Part model, mm, in its own coordinate system. A direction names the side the tool comes from. Coordinates: 2 decimals unless noted, no trailing zeros. Write each loop counter-clockwise with the first axis right and the second up, starting at its lowest first coordinate (ties: lowest second). Pieces come first, ordered by that corner, then holes. Notation, with made-up numbers: (6, -21.5) -> (10, -21.5) arc R16 ccw to (10, -1.5) -> close; hole circle Ø1 at (-33, -38.75). An arc over 180 degrees is marked (long way). One line per question, with ' | ' between items. Start each with the question number.
Item 1: Saw through at A-A (x = -82.5). List the corners of the cut face in (y, z), and give its area (3 significant figures).
Item 2: 3-axis set-ups, long thin cutter, end or side, ignore diameter. For faces 5 (the flat face through (-40, 42, 8)), 6 (the flat face through (40, 42, 8)), 7 (the cylindrical face through (88.849, 0.132, 3.254)), 8 (the flat face through (-1, 43, 15)): which of +Z, -Z, +X, -X, +Y, -Y reach the whole face in a straight line?
Item 3: Saw through at C-C (z = 12.5). Count the separate pieces of the cut face and the enclosed holes in it, and give its area (3 significant figures).
Item 4: Two-plate mould, pull along X, no slides. Class faces 1 (the flat face through (72, 0, 20)), 2 (the flat face through (-1, 0, 19.5)), 3 (the cylindrical face through (-85.8, 5.1, 13.4)), 4 (the flat face through (-105, 0, 10)): pulls with the +X half, pulls with the -X half, needs draft (parallel to the pull), parting line crosses it, or undercut.
Item 5: Saw through at D-D (x = 44). List the corners of the cut face in (y, z), and give its area (3 significant figures).
Item 6: Saw through at B-B (y = -6.5). List the corners of the cut face in (x, z).
Item 7: Pin check, flat tips, straight feed: pin 1 (13 mm diameter, centred on x = -82.5, y = 5, fed in from -Z); pin 2 (12 mm diameter, centred on y = 45.5, z = 6, fed in from -X); pin 3 (6.5 mm diameter, centred on x = -23, y = 6.5, fed in from +Z); pin 4 (21 mm diameter, centred on x = 82.5, y = 5, fed in from +Z). Stop position of each tip, or through.
Item 8: Probe probe 1 along Y at (x, z) = (82.5, 14.5); probe 2 along Y at (x, z) = (-25, 5.25); probe 3 along Y at (x, z) = (82.5, 1.5). List the from-to ranges inside material, lowest first. Write a range as [from, to].
from build123d import *

# Parameters (mm, degrees)
SKETCH1_W                                      = 210
SKETCH1_H                                      = 50
EXTRUDE1_DEPTH                                 = 20
CBORE_FOR_M6_HEX_HEAD_FLANGE_BOLT1_D           = 6.6
CBORE_FOR_M6_HEX_HEAD_FLANGE_BOLT1_CBORE_D     = 16
CBORE_FOR_M6_HEX_HEAD_FLANGE_BOLT1_CBORE_DEPTH = 6.6
CUT_EXTRUDE1_REACH                             = 52
SKETCH4_W                                      = 80
SKETCH4_H                                      = 0.5
M6_TAPPED_HOLE1_D                              = 5
SKETCH7_W                                      = 80
SKETCH7_H                                      = 35
EXTRUDE2_DEPTH                                 = 19.5
SKETCH8_W                                      = 80
SKETCH8_H                                      = 5
CUT_EXTRUDE2_DEPTH                             = 35
M6_TAPPED_HOLE2_D                              = 5


with BuildPart() as part:
    # Sketch1 → Extrude1 (new body)
    with BuildSketch(Plane.XY):
        Rectangle(SKETCH1_W, SKETCH1_H)
    extrude(amount=EXTRUDE1_DEPTH)

    # CBORE for M6 Hex Head Flange Bolt1 (through all)
    with Locations(Plane(origin=(0, 0, 0), x_dir=(-1, 0, 0), z_dir=(0, 0, -1))):
        with Locations((82.5, 5), (-82.5, 5)):
            CounterBoreHole(CBORE_FOR_M6_HEX_HEAD_FLANGE_BOLT1_D / 2, CBORE_FOR_M6_HEX_HEAD_FLANGE_BOLT1_CBORE_D / 2, CBORE_FOR_M6_HEX_HEAD_FLANGE_BOLT1_CBORE_DEPTH)

    # Sketch4 → Cut-Extrude1 (cut, up to next)
    with BuildSketch(Plane(origin=(0, 25, 0), x_dir=(1, 0, 0), z_dir=(0, 1, 0)), mode=Mode.PRIVATE) as cut_extrude1_sk1:
        with Locations((0, -19.75)):
            Rectangle(SKETCH4_W, SKETCH4_H)
    cut_extrude1_tool1 = extrude(cut_extrude1_sk1.sketch, amount=-CUT_EXTRUDE1_REACH, mode=Mode.PRIVATE) & part.part
    add(cut_extrude1_tool1.solids().sort_by_distance((0, 25, 19.75))[0], mode=Mode.SUBTRACT)

    # M6 Tapped Hole1 (through all)
    with Locations(Plane.XY.offset(19.5)):
        with Locations((-23, 6.5), (-23, -6.5), (23, 6.5), (23, -6.5)):
            Hole(M6_TAPPED_HOLE1_D / 2)

    # Sketch7 → Extrude2 (add)
    with BuildSketch(Plane.XY.offset(19.5)):
        with Locations((0, 42.5)):
            Rectangle(SKETCH7_W, SKETCH7_H)
    extrude(amount=-EXTRUDE2_DEPTH)

    # Sketch8 → Cut-Extrude2 (cut)
    with BuildSketch(Plane(origin=(0, 60, 0), x_dir=(1, 0, 0), z_dir=(0, 1, 0))):
        with Locations((0, -17.5)):
            Rectangle(SKETCH8_W, SKETCH8_H)
    extrude(amount=-CUT_EXTRUDE2_DEPTH, mode=Mode.SUBTRACT)

    # M6 Tapped Hole2 (through all)
    with Locations(Plane.XY.offset(15)):
        with Locations((-25, 46.359410027), (25, 46.359410027)):
            Hole(M6_TAPPED_HOLE2_D / 2)


solid = part.part
From the geometry:
1) outline: (-25, 0) -> (-3, 0) -> (-3, 6.6) -> (1.7, 6.6) -> (1.7, 20) -> (-25, 20) -> close; (8.3, 6.6) -> (13, 6.6) -> (13, 0) -> (25, 0) -> (25, 20) -> (8.3, 20) -> close | area: 806 mm2
2) face 5: +Z, -Z, -X, +Y | face 6: +Z, -Z, +X, +Y | face 7: -Z | face 8: +Z, +X, -X, +Y
3) separate pieces: 1 | enclosed holes: 8 | area: 13,100 mm2
4) face 1: needs draft | face 2: undercut | face 3: undercut | face 4: pulls with the -X half
5) outline: (-25, 0) -> (25, 0) -> (25, 20) -> (-25, 20) -> close | area: 1,000 mm2
6) outline: (-105, 0) -> (-25.5, 0) -> (-25.5, 19.5) -> (-40, 19.5) -> (-40, 20) -> (-105, 20) -> close; (-20.5, 0) -> (20.5, 0) -> (20.5, 19.5) -> (-20.5, 19.5) -> close; (25.5, 0) -> (105, 0) -> (105, 20) -> (40, 20) -> (40, 19.5) -> (25.5, 19.5) -> close
7) pin 1: z = 6.6 | pin 2: x = -40 | pin 3: z = 19.5 | pin 4: z = 20
8) probe 1: [-25, 1.7], [8.3, 25] | probe 2: [-25, -8], [-5, 5], [8, 43.86], [48.86, 60] | probe 3: [-25, -3], [13, 25]
